Verification items for the finished model (mm, model axes). Face numbers are marked on the shaded views. A direction names the side the tool comes from. Round coordinates to 2 decimals unless told otherwise and drop trailing zeros. Write each loop counter-clockwise with the first axis right and the second up, starting at its lowest first coordinate (ties: lowest second). Pieces come first, ordered by that corner, then holes. Notation, with made-up numbers: M 15,1 L 64,1 A22 ccw 64,35 Z; hole C 18.25,30 d7. An arc over 180 degrees is marked long. Answer in a Markdown table with one row per item. Add a question column.
1. Sectioned sample at D-D on y = -8. Record the cut outline in (x, z), plus the area to 3 significant figures.
2. Set-up check for the marked faces 4, 5, 6 and 7: record each of +Z, -Z, +X, -X, +Y, -Y from which the full face is reachable in a straight line by a thin tool's end or side.
3. Material ranges on probe 1 along Y at (x, z) = (22.5, 3.5); probe 2 along X at (y, z) = (18, 2); probe 3 along X at (y, z) = (-13, 5.75), recorded low to high.
4. Sectioned sample at B-B on y = 0. Record the cut outline in (x, z) (3 decimals), plus the area to 3 significant figures.
5. Sectioned sample at A-A on x = 22.5. Record the cut outline in (y, z).
6. Sectioned sample at C-C on x = 8. Record the cut outline in (y, z), plus the area to 3 significant figures.
7. Draft check along Y on the marked faces 1, 2 and 3. Enter one of: pulls with the +Y half, pulls with the -Y half, needs draft (parallel to the pull), parting line crosses it, or undercut.
8. Go/stop test with flat-tipped pins: pin 1 Ø2.5 at (x, z) = (-3.5, 2) entering from -Y; pin 2 Ø2.5 at (x, z) = (3, 4) entering from +Y; pin 3 Ø1.9 at (y, z) = (-21.5, 3) entering from -X. Record where each tip stops, or that it passes through.
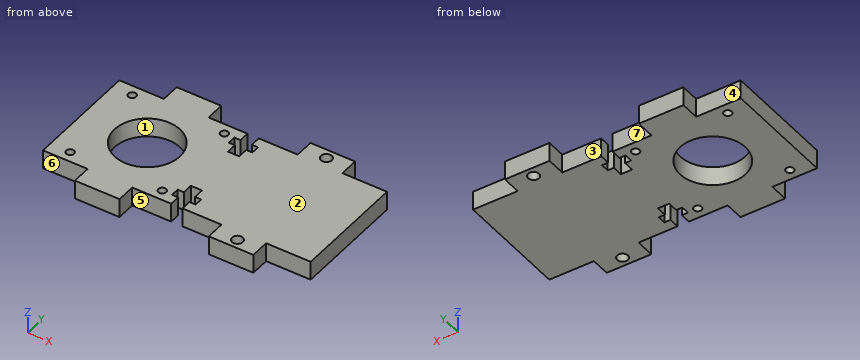
```python
from build123d import *

# Parameters (mm, degrees)
SKETCH1_W             = 90
SKETCH1_H             = 50.8
BOSS_EXTRUDE1_DEPTH   = 6.35
SKETCH2_R             = 7.9375
SKETCH2_W             = 15
SKETCH2_H             = 6.35
SKETCH2_W_2           = 30
CUT_EXTRUDE1_DEPTH    = 6.35
CUT_EXTRUDE3_DEPTH    = 53.062294417
SKETCH3_R             = 11
SKETCH3_R_2           = 1.3208
CUT_EXTRUDE2_DEPTH    = 53.062294417
F_6_CLEARANCE_HOLE1_D = 3.6576


with BuildPart() as part:
    # Sketch1 → Boss-Extrude1 (new body)
    with BuildSketch(Plane.XY):
        Rectangle(SKETCH1_W, SKETCH1_H)
    extrude(amount=BOSS_EXTRUDE1_DEPTH)

    # Sketch2 → Cut-Extrude1 (cut)
    with BuildSketch(Plane.XY.offset(6.35)):
        with Locations((-22.775, 0)):
            Circle(SKETCH2_R)
        with Locations((-37.5, -22.225)):
            Rectangle(SKETCH2_W, SKETCH2_H)
        with Locations((0, -22.225)):
            Rectangle(SKETCH2_W_2, SKETCH2_H)
        with Locations((37.5, -22.225)):
            Rectangle(SKETCH2_W, SKETCH2_H)
    cut_extrude1 = extrude(amount=-CUT_EXTRUDE1_DEPTH, mode=Mode.SUBTRACT)

    # Sketch9 → Cut-Extrude3 (cut, through all)
    with BuildSketch(Plane.XY.offset(6.35)):
        Polygon((-1.89865, -9.271), (1.89865, -9.271), (1.89865, -12.7714375), (3.96875, -12.7714375), (3.96875, -15.5495625), (1.89865, -15.5495625), (1.89865, -19.05), (-1.89865, -19.05), (-1.89865, -15.5495625), (-3.96875, -15.5495625), (-3.96875, -12.7714375), (-1.89865, -12.7714375), align=None)
    cut_extrude3 = extrude(amount=-CUT_EXTRUDE3_DEPTH, mode=Mode.SUBTRACT)

    # Mirror2: Cut-Extrude1, Cut-Extrude3 across plane
    add(cut_extrude1.mirror(Plane.ZX), mode=Mode.SUBTRACT)
    add(cut_extrude3.mirror(Plane.ZX), mode=Mode.SUBTRACT)

    # Sketch3 → Cut-Extrude2 (cut, through all)
    with BuildSketch(Plane.XY.offset(6.35)):
        with Locations((-22.775, 0)):
            Circle(SKETCH3_R)
        with Locations((-38.275, 15.5)):
            Circle(SKETCH3_R_2)
        with Locations((-7.275, 15.5)):
            Circle(SKETCH3_R_2)
        with Locations((-7.275, -15.5)):
            Circle(SKETCH3_R_2)
        with Locations((-38.275, -15.5)):
            Circle(SKETCH3_R_2)
    extrude(amount=-CUT_EXTRUDE2_DEPTH, mode=Mode.SUBTRACT)

    # #6 Clearance Hole1 (through all)
    with Locations(Plane.XY.offset(6.35)):
        with Locations((22.5, -22.225)):
            f_6_clearance_hole1 = Hole(F_6_CLEARANCE_HOLE1_D / 2)

    # Mirror3: #6 Clearance Hole1 across plane
    add(f_6_clearance_hole1.mirror(Plane.ZX), mode=Mode.SUBTRACT)


solid = part.part
```
Geometry check:
| question | item | result |
|---|---|---|
| 1 | outline | M -45,0 L -30.32,0 L -30.32,6.35 L -45,6.35 Z; M -15.23,0 L 45,0 L 45,6.35 L -15.23,6.35 Z |
| 1 | area | 476 mm2 |
| 2 | face 4 | +Z, -Z, -X, +Y |
| 2 | face 5 | +Z, -Z, -Y |
| 2 | face 6 | +Z, -Z, -X, -Y |
| 2 | face 7 | +Z, -Z, +Y |
| 3 | probe 1 | y = -25.4 to -24.05, -20.4 to 20.4, 24.05 to 25.4 |
| 3 | probe 2 | x = -45 to -1.9, 1.9 to 45 |
| 3 | probe 3 | x = -45 to -3.97, 3.97 to 45 |
| 4 | outline | M -45,0 L -33.775,0 L -33.775,6.35 L -45,6.35 Z; M -11.775,0 L 45,0 L 45,6.35 L -11.775,6.35 Z |
| 4 | area | 432 mm2 |
| 5 | outline | M -25.4,0 L -24.05,0 L -24.05,6.35 L -25.4,6.35 Z; M -20.4,0 L 20.4,0 L 20.4,6.35 L -20.4,6.35 Z; M 24.05,0 L 25.4,0 L 25.4,6.35 L 24.05,6.35 Z |
| 6 | outline | M -19.05,0 L 19.05,0 L 19.05,6.35 L -19.05,6.35 Z |
| 6 | area | 242 mm2 |
| 7 | face 1 | undercut |
| 7 | face 2 | needs draft |
| 7 | face 3 | pulls with the +Y half |
| 8 | pin 1 | stops at y = -19.05 |
| 8 | pin 2 | stops at y = 19.05 |
| 8 | pin 3 | stops at x = -30 |
